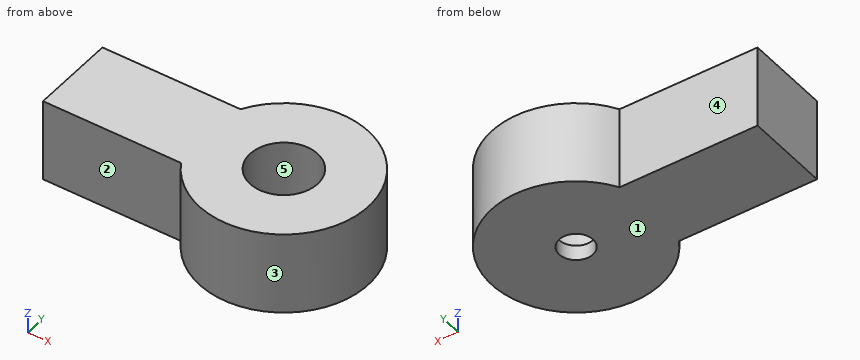
```python
from build123d import *

# Parameters (mm, degrees)
BOSS_EXTRUDE2_DEPTH = 12.446
SKETCH4_R           = 2.54
CUT_EXTRUDE1_DEPTH  = 13.446
SKETCH5_R           = 5.08
CUT_EXTRUDE2_DEPTH  = 10.16


with BuildPart() as part:
    # Sketch3 → Boss-Extrude2 (new body)
    with BuildSketch(Plane.XY):
        with BuildLine():
            Line((-10.998522628, -6.35), (-19.05, -6.35))
            Line((-19.05, -6.35), (-31.75, -6.35))
            Line((-31.75, -6.35), (-31.75, 6.35))
            Line((-31.75, 6.35), (-19.05, 6.35))
            Line((-19.05, 6.35), (-10.998522628, 6.35))
            ThreePointArc((-10.998522628, 6.35), (12.7, 0), (-10.998522628, -6.35))
        make_face()
    extrude(amount=BOSS_EXTRUDE2_DEPTH)

    # Sketch4 → Cut-Extrude1 (cut, through all)
    with BuildSketch(Plane(origin=(0, 0, 0), x_dir=(-1, 0, 0), z_dir=(0, 0, -1))):
        Circle(SKETCH4_R)
    extrude(amount=-CUT_EXTRUDE1_DEPTH, mode=Mode.SUBTRACT)

    # Sketch5 → Cut-Extrude2 (cut)
    with BuildSketch(Plane.XY.offset(12.446)):
        Circle(SKETCH5_R)
    extrude(amount=-CUT_EXTRUDE2_DEPTH, mode=Mode.SUBTRACT)


solid = part.part
```
Source: CAD feature listing. Evaluate the final solid. Frame: model axes, mm. Face numbers are marked on the shaded views. A direction names the side the tool comes from. Round coordinates to 2 decimals unless told otherwise and drop trailing zeros. Loops run counter-clockwise (first coordinate to the right, second up) from the corner with the lowest first, then second, coordinate; pieces in that order, holes last.
(1) Pull-direction query (X, two-part tool) for the marked faces 3, 4 and 5; classes: +X half, -X half, draft (parallel to the pull), parting line (faces both ways), or undercut.
From the geometry:
face 3: parting line
face 4: draft
face 5: undercut
(2) Section query A-A (x = 0). Output: boundary loops of the cut face in (y, z).
From the geometry:
outline: (-12.7, 0) - (-2.54, 0) - (-2.54, 2.29) - (-5.08, 2.29) - (-5.08, 12.45) - (-12.7, 12.45) - close; (2.54, 0) - (12.7, 0) - (12.7, 12.45) - (5.08, 12.45) - (5.08, 2.29) - (2.54, 2.29) - close
(3) Contact query for flat-ended pins moving along their axis: pin 1 Ø4 at (x, z) = (-8.5, 4.5) entering from +Y; pin 2 Ø6 at (x, y) = (-4.5, -0.5) entering from -Z; pin 3 Ø6.5 at (x, y) = (0, 0) entering from +Z; pin 4 Ø1.5 at (x, z) = (2.5, 4) entering from -Y. Output: stop coordinate, or through.
From the geometry:
pin 1: stops at y = 10.91
pin 2: stops at z = 0
pin 3: stops at z = 2.29
pin 4: stops at y = -12.58
(4) Access query for the marked faces 1 and 2. Directions: +Z, -Z, +X, -X, +Y, -Y. A direction counts if a zero-diameter tool reaches every point of the face in a straight line with its end or side. Return the directions, or none.
From the geometry:
face 1: -Z, +X, -X, +Y, -Y
face 2: +Z, -Z, -X, -Y
(5) Section query B-B (y = 0). Output: boundary loops of the cut face in (x, z).
From the geometry:
outline: (-31.75, 0) - (-2.54, 0) - (-2.54, 2.29) - (-5.08, 2.29) - (-5.08, 12.45) - (-31.75, 12.45) - close; (2.54, 0) - (12.7, 0) - (12.7, 12.45) - (5.08, 12.45) - (5.08, 2.29) - (2.54, 2.29) - close
(6) Section query C-C (z = 7.75). Output: boundary loops of the cut face in (x, y), and give its area (3 significant figures).
From the geometry:
outline: (-31.75, -6.35) - (-11, -6.35) arc R12.7 ccw (long way) to (-11, 6.35) - (-31.75, 6.35) - close; hole circle Ø10.16 at (0, 0)
area: 675 mm2
(7) Material intervals for probe 1 along Y at (x, z) = (-15, 1); probe 2 along X at (y, z) = (2, 11.75); probe 3 along X at (y, z) = (0.25, 9.75), sorted ascending.
From the geometry:
probe 1: y = -6.35 to 6.35
probe 2: x = -31.75 to -4.67, 4.67 to 12.54
probe 3: x = -31.75 to -5.07, 5.07 to 12.7
(8) Section query D-D (x = -21). Output: boundary loops of the cut face in (y, z).
From the geometry:
outline: (-6.35, 0) - (6.35, 0) - (6.35, 12.45) - (-6.35, 12.45) - close
